```python
from build123d import *

# Parameters (mm, degrees)
SKETCH4_W            = 90
SKETCH4_H            = 60
BOSS_EXTRUDE13_DEPTH = 32
BOSS_EXTRUDE14_DEPTH = 54
SKETCH4_30_W         = 24
SKETCH4_30_H         = 20
BOSS_EXTRUDE16_DEPTH = 33
BOSS_EXTRUDE17_DEPTH = 16
SKETCH5_W            = 30
SKETCH5_H            = 23
CUT_EXTRUDE2_DEPTH   = 100
CUT_EXTRUDE3_DEPTH   = 100
CUT_EXTRUDE6_DEPTH   = 100


with BuildPart() as part:
    # Sketch4 → Boss-Extrude13 (new body)
    with BuildSketch(Plane(origin=(0, 0, 0), x_dir=(1, 0, 0), z_dir=(0, 1, 0))):
        with Locations((-31.3432161, 7.554270448)):
            Rectangle(SKETCH4_W, SKETCH4_H)
    extrude(amount=-BOSS_EXTRUDE13_DEPTH)

    # Sketch4_27 → Boss-Extrude14 (add)
    with BuildSketch(Plane(origin=(0, 0, 0), x_dir=(1, 0, 0), z_dir=(0, 1, 0))):
        with BuildLine():
            ThreePointArc((-54.256094575, 17.554270448), (-55.815873922, 12.662011545), (-56.3432161, 7.554270458))
            ThreePointArc((-56.3432161, 7.554270458), (-55.815873924, 2.446529361), (-54.256094575, -2.445729552))
            Line((-54.256094575, -2.445729552), (-43.3432161, -2.445729552))
            Line((-43.3432161, -2.445729552), (-43.3432161, 17.554270448))
            Line((-43.3432161, 17.554270448), (-54.256094575, 17.554270448))
        make_face()
        with BuildLine():
            ThreePointArc((-8.430337625, -2.445729552), (-6.870558277, 2.446529356), (-6.3432161, 7.554270448))
            ThreePointArc((-6.3432161, 7.554270448), (-6.870558277, 12.66201154), (-8.430337625, 17.554270448))
            Line((-8.430337625, 17.554270448), (-19.3432161, 17.554270448))
            Line((-19.3432161, 17.554270448), (-19.3432161, -2.445729552))
            Line((-19.3432161, -2.445729552), (-8.430337625, -2.445729552))
        make_face()
    extrude(amount=BOSS_EXTRUDE14_DEPTH)

    # Sketch4_30 → Boss-Extrude16 (add)
    with BuildSketch(Plane(origin=(0, 0, 0), x_dir=(1, 0, 0), z_dir=(0, 1, 0))):
        with Locations((-31.3432161, 7.554270448)):
            Rectangle(SKETCH4_30_W, SKETCH4_30_H)
    extrude(amount=BOSS_EXTRUDE16_DEPTH)

    # Sketch4_31 → Boss-Extrude17 (add)
    with BuildSketch(Plane(origin=(0, 0, 0), x_dir=(1, 0, 0), z_dir=(0, 1, 0))):
        with BuildLine():
            Line((-43.3432161, -2.445729552), (-54.256094575, -2.445729552))
            ThreePointArc((-54.256094575, -2.445729552), (-31.3432161, -17.445729552), (-8.430337625, -2.445729552))
            Line((-8.430337625, -2.445729552), (-19.3432161, -2.445729552))
            Line((-19.3432161, -2.445729552), (-43.3432161, -2.445729552))
        make_face()
        with BuildLine():
            ThreePointArc((-8.430337625, 17.554270448), (-31.3432161, 32.554270448), (-54.256094575, 17.554270448))
            Line((-54.256094575, 17.554270448), (-43.3432161, 17.554270448))
            Line((-43.3432161, 17.554270448), (-19.3432161, 17.554270448))
            Line((-19.3432161, 17.554270448), (-8.430337625, 17.554270448))
        make_face()
    extrude(amount=BOSS_EXTRUDE17_DEPTH)

    # Sketch5 → Cut-Extrude2 (cut)
    with BuildSketch(Plane.ZY.offset(76.3432161)):
        with Locations((-7.554270448, -20.5)):
            Rectangle(SKETCH5_W, SKETCH5_H)
    extrude(amount=-CUT_EXTRUDE2_DEPTH, mode=Mode.SUBTRACT)

    # Sketch7 → Cut-Extrude3 (cut)
    with BuildSketch(Plane.XY):
        Polygon((-56.214551836, 0), (-76.3432161, 0), (-76.3432161, -24), align=None)
        Polygon((13.6567839, 0), (13.6567839, -24), (-6.3432161, 0), align=None)
    extrude(amount=-CUT_EXTRUDE3_DEPTH, mode=Mode.SUBTRACT)

    # Sketch7_4 → Cut-Extrude6 (cut)
    with BuildSketch(Plane.XY):
        Polygon((13.6567839, 0), (13.6567839, -24), (-6.3432161, 0), align=None)
        Polygon((-56.214551836, 0), (-76.3432161, 0), (-76.3432161, -24), align=None)
    extrude(amount=CUT_EXTRUDE6_DEPTH, mode=Mode.SUBTRACT)


solid = part.part
```
Part model, mm, in its own coordinate system. A direction names the side the tool comes from. Give positions to 0.01 mm unless a question says otherwise; leave off trailing zeros. Write each loop counter-clockwise with the first axis right and the second up, starting at its lowest first coordinate (ties: lowest second). Pieces come first, ordered by that corner, then holes. Notation, with made-up numbers: (32, 61) -> (43, 61) arc R21 cw to (43, 85) -> close; hole circle Ø7 at (-36.75, 8). An arc over 180 degrees is marked (long way). Put each result on its own line as item: value. Start each with the question number.
Item 1: Cut at A-A (x = 5.5). List the corners of the cut face in (y, z), then the cut area to 3 significant figures.
Item 2: Pin check, flat tips, straight feed: pin 1 Ø11.5 at (x, y) = (-34.5, 38.5) entering from +Z; pin 2 Ø10 at (y, z) = (47, -12) entering from -X; pin 3 Ø15 at (x, z) = (-28, 5.5) entering from +Y; pin 4 Ø10 at (y, z) = (42.5, 10.5) entering from -X. Stop position of each tip, or through.
Item 3: Cut at B-B (y = -13). List the corners of the cut face in (x, z).
Item 4: Pull direction X, two halves, no side cores. Call faces 6 (the face through (-32, 33, -8)), 7 (the face through (-19.343, 43, -8)), 8 (the face through (-76.343, -28, -30)), 9 (the face through (-32, -9, -8)): pulls with the +X half, pulls with the -X half, needs draft (parallel to the pull), parting line crosses it, or undercut.
Item 5: Wall check: L1, parallel to Z at x = -17, y = -27; L2, parallel to X at y = 34, z = -8.5; L3, parallel to Y at x = -30, z = -34.5. Give the ranges that are in metal, low to high. Write a range as [from, to].
Item 6: Cut at C-C (y = 22). List the corners of the cut face in (x, z), then the cut area to 3 significant figures.
Item 7: Which spindle directions (+Z, -Z, +X, -X, +Y, -Y) get a long thin tool onto all of the face, cutting with end or side? Do faces 1 (the face through (-32, 16, 8)), 2 (the face through (-32, -21, -22.554)), 3 (the face through (-30, 0, 18)), 4 (the face through (-50, 54, -8)), 5 (the face through (-32, 16, -23)). Say none if no direction does.
Item 8: Cut at D-D (z = 4.5). List the corners of the cut face in (x, y).
Answer list:
1. outline: (-32, -37.55) -> (-14.21, -37.55) -> (-14.21, -22.55) -> (-32, -22.55) -> close; (-32, 7.45) -> (-14.21, 7.45) -> (-14.21, 22.45) -> (-32, 22.45) -> close
1. area: 534 mm2
2. pin 1: stops at z = 2.45
2. pin 2: stops at x = -56.34
2. pin 3: stops at y = 33
2. pin 4: passes through
3. outline: (-67.12, -37.55) -> (4.49, -37.55) -> (4.49, -22.55) -> (-67.12, -22.55) -> close; (-67.12, 7.45) -> (4.49, 7.45) -> (4.49, 22.45) -> (-67.12, 22.45) -> close
4. face 6: undercut
4. face 7: undercut
4. face 8: pulls with the -X half
4. face 9: needs draft
5. L1: z = [-37.55, -22.55], [7.45, 22.45]
5. L2: x = [-56.33, -43.34], [-19.34, -6.36]
5. L3: y = [-32, 0]
6. outline: (-54.26, -17.55) -> (-8.43, -17.55) arc R25 ccw to (-8.43, 2.45) -> (-54.26, 2.45) arc R25 ccw to start
6. area: 973 mm2
7. face 1: +Z, +X, -X, +Y
7. face 2: +X, -X, -Y
7. face 3: +Z, +Y
7. face 4: +Z, -Z, +X, -X, +Y
7. face 5: -Z, +X, -X, +Y
8. outline: (-63.76, -9) -> (1.16, -9) -> (-6.34, 0) -> (-9.44, 0) -> (-9.44, 16) -> (-53.25, 16) -> (-53.25, 0) -> (-56.21, 0) -> close
